Read the model definition and answer for the solid it produces. Units are mm, in the model's axes. A direction names the side the tool comes from. Round coordinates to 2 decimals unless told otherwise and drop trailing zeros. Order: outer loops, then holes, each group sorted by start corner. A loop starts at its lowest first (then second) coordinate and runs counter-clockwise, first axis right, second up. Notation, with made-up numbers: M 6,54.5 L 64,54.5 A18 ccw 64,64.5 Z; hole C -8,43 d3. An arc over 180 degrees is marked long. Answer as CSV lines item,"result".
Autodesk Inventor part; units mm, degrees
ref_plane "YZ Plane" through (0, 0, 0) normal (1, 0, 0) x (0, 1, 0)
ref_plane "XZ Plane" through (0, 0, 0) normal (0, 1, 0) x (-1, 0, 0)
ref_plane "XY Plane" through (0, 0, 0) normal (0, 0, 1) x (1, 0, 0)
sketch "Skizze1" plane through (0, 0, 0) normal (0, 0, 1) x (1, 0, 0)
  line L0 (25.5223, 16.961) -> (0, 12)
  line L1 (0, 12) -> (0, 0)
  line L2 (0, 0) -> (25.0305, -7.0339)
  line L3 (25.0305, -7.0339) -> (25.5223, 16.961)
  line L4 (-3, 14.473) -> (28.5978, 20.615)
  line L5 (28.5978, 20.615) -> (27.9504, -10.9707)
  line L6 (27.9504, -10.9707) -> (-3, -2.2732)
  line L7 (-3, -2.2732) -> (-3, 14.473)
  dimension "d0" = 26
  dimension "d1" = 12
  dimension "d3" = 26
  dimension "d4" = 24
  dimension "d7" = 101
  dimension "d8" = 77.826
  dimension "d9" = 3
  dimension "d10" = 3
  dimension "d11" = 3
  dimension "d12" = 3
extrude "Extrusion1" add sketch "Skizze1" along normal blind 150
sketch "Skizze3" plane through (0, 0, 0) normal (0, 1, 0) x (-1, 0, 0)
  line L0 (3, 0) -> (3, 150) construction
  line L1 (-27.9504, 0) -> (-28.5978, 0) construction
  line L2 (-28.5978, 0) -> (-28.5978, 150) construction
  line L3 (-27.9504, 150) -> (-28.5978, 150) construction
  line L4 (-27.9504, 0) -> (-27.9504, 150) construction
  line L5 (3, 0) -> (-28.5978, 6.7163)
  line L6 (-28.5978, 6.7163) -> (-28.5978, 0)
  line L7 (3, 150) -> (-28.5978, 140.9395)
  line L8 (-28.5978, 150) -> (-28.5978, 140.9395)
  line L9 (3, 150) -> (-27.9504, 150)
  line L10 (-28.5978, 150) -> (3, 150)
  line L11 (-27.9504, 0) -> (-28.5978, 0)
  line L12 (-28.5978, 0) -> (3, 0)
  point P0 (0, 0)
  dimension "d19" = 78
  dimension "d20" = 74
  dimension "d25" = 150
extrude "Extrusion2" cut sketch "Skizze3" along normal mid plane 149
fillet "Rundung1" radius 3 4 edges at (-3, -2.2732, 75) (27.9504, -10.9707, 73.8519) (-3, 14.473, 75) (28.5978, 20.615, 73.8279)
fillet "Rundung1" radius 1 4 edges at (25.5223, 16.961, 73.942) (25.0305, -7.0339, 73.9602) (0, 0, 74.8887) (0, 12, 74.8887)
equation "\"d10\" = d9"
equation "\"d11\" = d9"
equation "\"d12\" = d9"
properties part number "handle_body_final"
Item 1: A cutting plane is placed at A-A, the plane z = 18.5. Determine the outline of the cut face in (x, y), and give its area (3 significant figures).
Ans:
outline,"M -3,0 A3 ccw -0.81,-2.89 L 24.22,-9.92 A3 ccw 28.03,-7.1 L 28.52,16.9 A3 ccw 24.95,19.91 L -0.57,14.94 A3 ccw -3,12 Z; hole M 0,0.76 A1 ccw 0.73,-0.2 L 23.79,-6.68 A1 ccw 25.06,-5.74 L 25.5,15.72 A1 ccw 24.31,16.72 L 0.81,12.16 A1 ccw 0,11.18 Z"
area,"293 mm2"
Item 2: Find the intervals of material crossed by probe 1 along X at (y, z) = (6, 120); probe 2 along X at (y, z) = (0.5, 51); probe 3 along Y at (x, z) = (1.5, 116.5), in increasing order. Write a range as [from, to].
Ans:
probe 1,"[-3, 0], [25.3, 28.3]"
probe 2,"[-3, 0.03], [25.18, 28.19]"
probe 3,"[-3.54, -0.42], [12.29, 15.35]"
Item 3: Flat-ended cylindrical pins translate along their axes: pin 1 (6 mm diameter, centred on x = 4, z = 83, fed in from +Y); pin 2 (1.5 mm diameter, centred on x = 9, y = -3.5, fed in from +Z); pin 3 (8 mm diameter, centred on x = 10, z = 16, fed in from +Y). Find the tip coordinate at first contact, or state that the pin passes through.
Ans:
pin 1,"y = 16.42"
pin 2,"z = 146.77"
pin 3,"y = 17.78"
Item 4: A cutting plane is placed at C-C, the plane x = 13.5. Determine the outline of the cut face in (y, z).
Ans:
outline,"M -6.91,3.51 L -3.79,3.51 L -3.79,145.27 L -6.91,145.27 Z; M 14.62,3.51 L 17.68,3.51 L 17.68,145.27 L 14.62,145.27 Z"
Item 5: A cutting plane is placed at B-B, the plane y = 7. Determine the outline of the cut face in (x, z).
Ans:
outline,"M -3,0 L 0,0.64 L 0,149.14 L -3,150 Z; M 25.32,6.02 L 28.32,6.66 L 28.32,141.02 L 25.32,141.88 Z"
Item 6: A tool of negligible diameter and unlimited length cuts with its end or side. For faces 1 (the face through (12.722, 14.473, 73.822)), 2 (the face through (-2.4, -1.8, 76.1)), from which of +Z, -Z, +X, -X, +Y, -Y can it reach the whole face along a straight path? Write none if from no direction.
Ans:
face 1,"+Z, -Z"
face 2,"+Z, -Z, -X, -Y"
